```python
from build123d import *

# Parameters (mm, degrees)
SKETCH_1_W          = 40
SKETCH_1_H          = 12
EXTRUDE_1_DEPTH     = 8
SKETCH_2_W          = 19.7
SKETCH_2_H          = 8.5
CUT_EXTRUDE_1_DEPTH = 8
SKETCH_3_R          = 1
CUT_EXTRUDE_2_DEPTH = 8
SKETCH_4_R          = 1.75
CUT_EXTRUDE_3_DEPTH = 10


with BuildPart() as part:
    # 스케치1 → 보스-돌출1 (new body)
    with BuildSketch(Plane(origin=(0, 0, 0), x_dir=(1, 0, 0), z_dir=(0, 1, 0))):
        Rectangle(SKETCH_1_W, SKETCH_1_H)
    extrude(amount=EXTRUDE_1_DEPTH)

    # 스케치2 → 컷-돌출1 (cut)
    with BuildSketch(Plane(origin=(0, 8, 0), x_dir=(1, 0, 0), z_dir=(0, 1, 0))):
        Rectangle(SKETCH_2_W, SKETCH_2_H)
    extrude(amount=-CUT_EXTRUDE_1_DEPTH, mode=Mode.SUBTRACT)

    # 스케치3 → 컷-돌출2 (cut)
    with BuildSketch(Plane(origin=(0, 8, 0), x_dir=(1, 0, 0), z_dir=(0, 1, 0))):
        with Locations((-11.7, 3.3)):
            Circle(SKETCH_3_R)
        with Locations((11.7, -3.3)):
            Circle(SKETCH_3_R)
    extrude(amount=-CUT_EXTRUDE_2_DEPTH, mode=Mode.SUBTRACT)

    # 스케치4 → 컷-돌출3 (cut)
    with BuildSketch(Plane(origin=(0, 8, 0), x_dir=(1, 0, 0), z_dir=(0, 1, 0))):
        with Locations((-17, 0)):
            Circle(SKETCH_4_R)
        with Locations((17, 0)):
            Circle(SKETCH_4_R)
    extrude(amount=-CUT_EXTRUDE_3_DEPTH, mode=Mode.SUBTRACT)


solid = part.part
```
For this review, take the finished solid that the model builds, in its own axes (mm). A direction names the side the tool comes from. Round coordinates to 2 decimals unless told otherwise and drop trailing zeros. Write each loop counter-clockwise with the first axis right and the second up, starting at its lowest first coordinate (ties: lowest second). Pieces come first, ordered by that corner, then holes. Notation, with made-up numbers: (1.5, 88.5) -> (30.5, 88.5) arc R19 cw to (30.5, 105.5) -> close; hole circle Ø6 at (73, 64). An arc over 180 degrees is marked (long way). Use one line per item in the form item = value.
1) To check wall thickness, follow L1, parallel to X at y = 6.25, z = 3.3; L2, parallel to X at y = 4, z = 0; L3, parallel to X at y = 6, z = -3.3. State the ranges of each line that lie inside material, in increasing order. Write a range as from..to.
Found:
L1 = -20..-9.85, 9.85..10.7, 12.7..20
L2 = -20..-18.75, -15.25..-9.85, 9.85..15.25, 18.75..20
L3 = -20..-12.7, -10.7..-9.85, 9.85..20
2) Take a section at C-C, the plane y = 1.25. Write out the cut boundary in (x, z).
Found:
outline = (-20, -6) -> (20, -6) -> (20, 6) -> (-20, 6) -> close; hole circle Ø3.5 at (-17, 0); hole circle Ø2 at (-11.7, -3.3); hole (-9.85, -4.25) -> (9.85, -4.25) -> (9.85, 4.25) -> (-9.85, 4.25) -> close; hole circle Ø2 at (11.7, 3.3); hole circle Ø3.5 at (17, 0)
3) Take a section at A-A, the plane x = -2.5. Write out the cut boundary in (y, z), and give its area (3 significant figures).
Found:
outline = (0, -6) -> (8, -6) -> (8, -4.25) -> (0, -4.25) -> close; (0, 4.25) -> (8, 4.25) -> (8, 6) -> (0, 6) -> close
area = 28.0 mm2
4) Mouldability with a two-part tool opening along Z and no side actions: class faces 1 (the cylindrical face through (15.71, 4.06, -1.18)), 2 (the flat face through (20, 4, 0)), 3 (the flat face through (0, 4, 6)) as +Z half, -Z half, draft (parallel to the pull), parting line (faces both ways), or undercut.
Found:
face_1 = undercut
face_2 = draft
face_3 = +Z half
5) Tool access review of faces 4 (the flat face through (-9.85, 4, 0)), 5 (the flat face through (-20, 4, 0)): name each direction out of +Z, -Z, +X, -X, +Y, -Y from which nothing blocks a thin tool from reaching the whole face with its end or side.
Found:
face_4 = +Y, -Y
face_5 = +Z, -Z, -X, +Y, -Y
6) Take a section at D-D, the plane x = 11.7. Write out the cut boundary in (y, z).
Found:
outline = (0, -6) -> (8, -6) -> (8, 2.3) -> (0, 2.3) -> close; (0, 4.3) -> (8, 4.3) -> (8, 6) -> (0, 6) -> close
7) Clearance check with a flat-ended pin moving along its axis: pin 1 (1 mm diameter, centred on x = 15, z = -1.5, fed in from -Y). State where the tip first meets the part, or that it passes through.
Found:
pin_1 = 0
8) Take a section at B-B, the plane z = -3.3. Write out the cut boundary in (x, y).
Found:
outline = (-20, 0) -> (-12.7, 0) -> (-12.7, 8) -> (-20, 8) -> close; (-10.7, 0) -> (-9.85, 0) -> (-9.85, 8) -> (-10.7, 8) -> close; (9.85, 0) -> (20, 0) -> (20, 8) -> (9.85, 8) -> close
